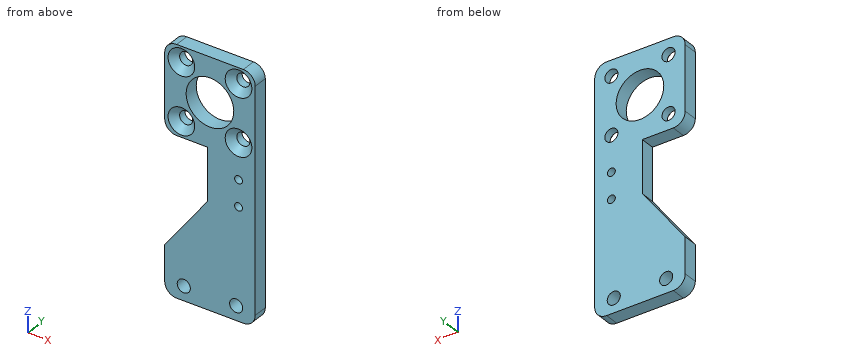
```python
from build123d import *

# Parameters (mm, degrees)
SKETCH_1_W                   = 38
SKETCH_1_H                   = 103
EXTRUDE_1_DEPTH              = 3
CUT_EXTRUDE_1_DEPTH          = 56.220014488
SKETCH_3_R                   = 10
CUT_EXTRUDE_2_DEPTH          = 56.220014488
HOLE_WIZARD_M5_1_D           = 5.5
HOLE_WIZARD_M5_1_CSINK_D     = 11.2
HOLE_WIZARD_M5_1_CSINK_ANGLE = 90
M4X0_7_1_D                   = 3.3
M4X0_7_1_DEPTH               = 10.1
M4X0_7_1_TIP                 = 0.991420021
SKETCH_8_R                   = 2.75
CUT_EXTRUDE_3_DEPTH          = 56.220014488
FILLET_1_R                   = 5


with BuildPart() as part:
    # 草图1 → 凸台-拉伸1 (new, symmetric)
    with BuildSketch(Plane(origin=(0, 0, 0), x_dir=(1, 0, 0), z_dir=(0, 1, 0))):
        Rectangle(SKETCH_1_W, SKETCH_1_H)
    extrude(amount=EXTRUDE_1_DEPTH, both=True)

    # 草图2 → 切除-拉伸1 (cut, through all)
    with BuildSketch(Plane(origin=(0, 3, 0), x_dir=(1, 0, 0), z_dir=(0, 1, 0))):
        Polygon((-19, -14.5), (-1, -14.5), (-1, 7.5), (-19, 31.5), align=None)
    extrude(amount=-CUT_EXTRUDE_1_DEPTH, mode=Mode.SUBTRACT)

    # 草图3 → 切除-拉伸2 (cut, through all)
    with BuildSketch(Plane(origin=(0, 3, 0), x_dir=(1, 0, 0), z_dir=(0, 1, 0))):
        with Locations(Location((0, -33, 0), (0, 0, 270))):
            Circle(SKETCH_3_R)
    extrude(amount=-CUT_EXTRUDE_2_DEPTH, mode=Mode.SUBTRACT)

    # M5 六角凹锥坑螺钉的锥形沉头孔1 (through all)
    with Locations(Plane.XZ.offset(3)):
        with Locations((12, 45), (-12, 45), (-12, 21), (12, 21)):
            CounterSinkHole(HOLE_WIZARD_M5_1_D / 2, HOLE_WIZARD_M5_1_CSINK_D / 2, counter_sink_angle=HOLE_WIZARD_M5_1_CSINK_ANGLE)

    # M4x0.7 螺纹孔1
    with Locations(Plane(origin=(0, 3, 0), x_dir=(-1, 0, 0), z_dir=(0, 1, 0))):
        with Locations((-12, -5), (-12, 6)):
            Hole(M4X0_7_1_D / 2, depth=M4X0_7_1_DEPTH)
            with Locations((0, 0, -(M4X0_7_1_DEPTH + M4X0_7_1_TIP / 2))):  # 118° drill point
                Cone(0, M4X0_7_1_D / 2, M4X0_7_1_TIP, mode=Mode.SUBTRACT)

    # 草图8 → 切除-拉伸3 (cut, through all)
    with BuildSketch(Plane(origin=(0, 3, 0), x_dir=(1, 0, 0), z_dir=(0, 1, 0))):
        with Locations(Location((-11, 45.5, 0), (0, 0, 270))):
            Circle(SKETCH_8_R)
        with Locations(Location((11, 45.5, 0), (0, 0, 270))):
            Circle(SKETCH_8_R)
    extrude(amount=-CUT_EXTRUDE_3_DEPTH, mode=Mode.SUBTRACT)

    # 圆角1
    fillet_1_edges = [part.edges().sort_by_distance(p)[0] for p in [
        (-19, 0, 14.5),
        (-19, 0, -51.5),
        (19, 0, -51.5),
        (19, 0, 51.5),
        (-19, 0, 51.5),
    ]]
    fillet(fillet_1_edges, radius=FILLET_1_R)


solid = part.part
```
Can you work these out from the model? Positions are in its coordinate system, mm. Round coordinates to 2 decimals unless told otherwise and drop trailing zeros. Order: outer loops, then holes, each group sorted by start corner. A loop starts at its lowest first (then second) coordinate and runs counter-clockwise, first axis right, second up.
(1) If we section it at A-A (z = 6): Please give me the cut outline in (x, y).
Results are:
outline: (-1, -3) - (10.35, -3) - (10.35, 3) - (-1, 3) - close; (13.65, -3) - (19, -3) - (19, 3) - (13.65, 3) - close
(2) If we section it at D-D (y = 0.75): Count the separate pieces of the cut face and the enclosed holes in it, plus the area to 3 significant figures.
Results are:
separate pieces: 1
enclosed holes: 9
area: 2,800 mm2
(3) I'm going to push flat-ended pins straight in: pin 1 (7 mm diameter, centred on x = 12, z = 21, fed in from -Y); pin 2 (1.8 mm diameter, centred on y = 0, z = 2.5, fed in from -X). Where does each tip first touch, or does it pass through?
Results are:
pin 1: stops at y = -0.9
pin 2: stops at x = -1
(4) If I drill on L1, parallel to X at y = 1.65, z = 45; L2, parallel to Z at x = -14, y = 0.75; L3, parallel to Z at x = -14.5, y = 2.5, over which ranges is the centre line in solid material (lowest first)?
Results are:
L1: x = -19 to -14.75, -9.25 to 9.25, 14.75 to 19
L2: z = -51.5 to -24.83, 14.5 to 19.11, 22.89 to 43.11, 46.89 to 51.5
L3: z = -51.47 to -25.5, 14.53 to 19.85, 22.15 to 43.85, 46.15 to 51.47
(5) If we section it at B-B (x = 0): Please give me the cut outline in (y, z), plus the area to 3 significant figures.
Results are:
outline: (-3, -51.5) - (3, -51.5) - (3, 23) - (-3, 23) - close; (-3, 43) - (3, 43) - (3, 51.5) - (-3, 51.5) - close
area: 498 mm2
(6) If we section it at C-C (z = -45.5): Please give me the cut outline in (x, y), plus the area to 3 significant figures.
Results are:
outline: (-19, -3) - (-13.75, -3) - (-13.75, 3) - (-19, 3) - close; (-8.25, -3) - (8.25, -3) - (8.25, 3) - (-8.25, 3) - close; (13.75, -3) - (19, -3) - (19, 3) - (13.75, 3) - close
area: 162 mm2
